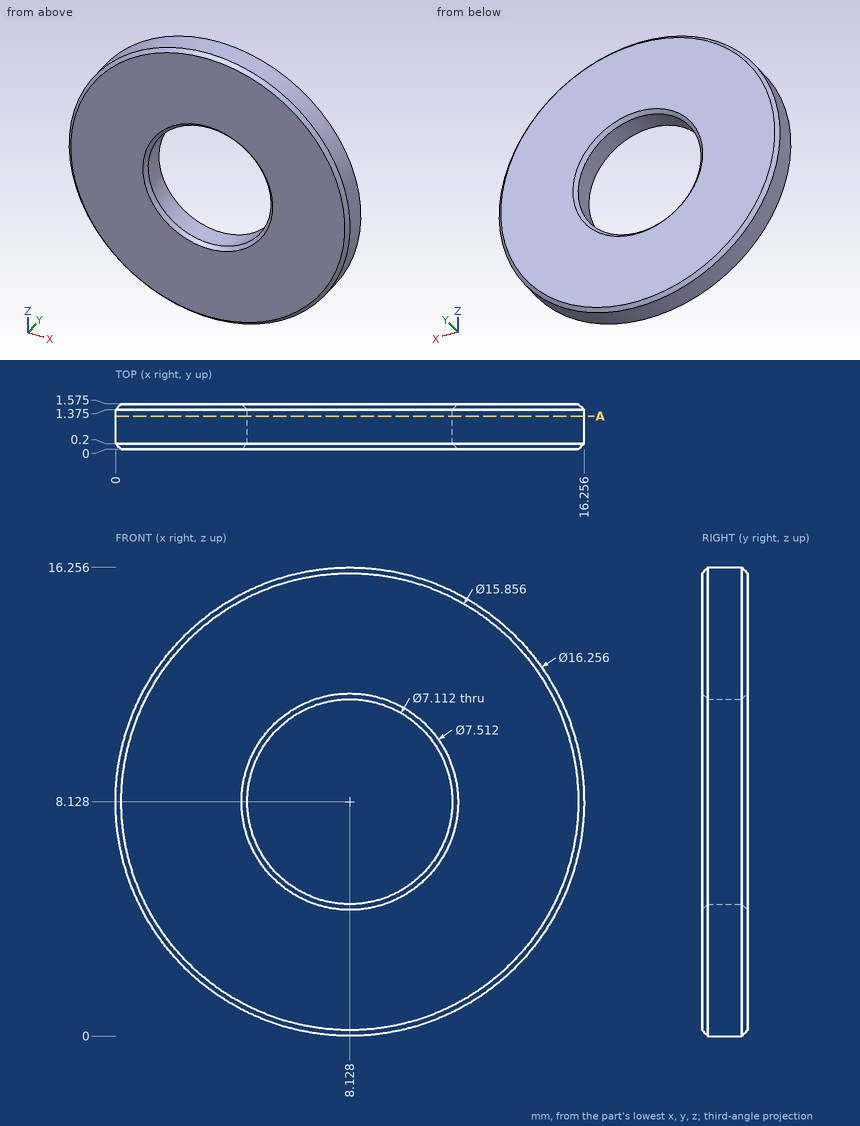
For this review, use the dimensioned drawing (mm, ordinates from the lowest corner) and the shaded views. Round coordinates to 2 decimals unless told otherwise and drop trailing zeros. Write each loop counter-clockwise with the first axis right and the second up, starting at its lowest first coordinate (ties: lowest second). Pieces come first, ordered by that corner, then holes. Notation, with made-up numbers: (41, 64.5) - (60, 64.5) arc R13 ccw to (60, 88.5) - close; hole circle Ø7 at (-16.75, 57.25). An arc over 180 degrees is marked (long way). Answer as a JSON object with one key per item and string values.
1. To check wall thickness, follow line 1 along Z through (x, y) = (8, 1.35) (1 decimal); line 2 along Z through (x, y) = (7.75, 0.7); line 3 along X through (y, z) = (0.8, 9) (1 decimal). State the ranges of each line that lie inside material, in increasing order.
Response values:
{"line 1": "z = 0 to 4.6, 11.7 to 16.3", "line 2": "z = 0.01 to 4.59, 11.66 to 16.25", "line 3": "x = 0 to 4.7, 11.6 to 16.2"}
2. We need section A-A on y = 1.15. Give the boundary of the cut face in (x, z), then the cut area to 3 significant figures.
Response values:
{"outline": "circle Ø16.26 at (8.13, 8.13); hole circle Ø7.11 at (8.13, 8.13)", "area": "168 mm2"}
3. For pin 1 Ø4 at (x, z) = (5.5, 3.5) entering from -Y; pin 2 Ø6.5 at (x, z) = (8.128, 8.128) entering from -Y, all flat-tipped, find the tip position at first contact; note any pin that passes through.
Response values:
{"pin 1": "stops at y = 0", "pin 2": "passes through"}
